Part model, mm, in its own coordinate system. A direction names the side the tool comes from. Round coordinates to 2 decimals unless told otherwise and drop trailing zeros. Write each loop counter-clockwise with the first axis right and the second up, starting at its lowest first coordinate (ties: lowest second). Pieces come first, ordered by that corner, then holes. Notation, with made-up numbers: (69.25, -13) -> (93.25, -13) arc R19 ccw to (93.25, 17) -> close; hole circle Ø1 at (20, 39). An arc over 180 degrees is marked (long way). Use CSV: the item, a comma, the result in double quotes. Start each with the question number.
(1) Saw through at D-D (x = -0.25). Give the cut face in (y, z).
(2) Saw through at A-A (x = 7.5). Give the cut face in (y, z), plus the area to 3 significant figures.
(3) Saw through at B-B (z = 0). Give the cut face in (x, y), plus the area to 3 significant figures.
(4) Which spindle directions (+Z, -Z, +X, -X, +Y, -Y) get a long thin tool onto all of the face, cutting with end or side? Do faces 5 (the flat face through (-11.5, 0.3, -4.3)), 6 (the flat face through (-12.5, 0.5, 0.1)). Say none if no direction does.
(5) Two-plate mould, pull along X, no slides. Class faces 1 (the cylindrical face through (-12.215, 0.507, 4.699)), 2 (the flat face through (-10, 0.3, -4.3)), 3 (the flat face through (10, 0.3, -4.3)), 4 (the flat face through (12.5, 0.5, -0.1)): released by +X, released by -X, zero draft, split by the parting line, or undercut.
(6) Probe line 1 (X direction, y = 0.65, z = 0); line 2 (Z direction, x = 7.5, y = 1.05); line 3 (X direction, y = 1.55, z = 0). List the from-to ranges inside material, lowest first. Write a range as [from, to].
Autodesk Inventor part; units mm, degrees
ref_plane "Work Plane1" through (0, 5, 0) normal (0, -1, 0) x (1, 0, 0)
ref_plane "YZ Plane" through (0, 0, 0) normal (1, 0, 0) x (0, 1, 0)
ref_plane "XZ Plane" through (0, 0, 0) normal (0, 1, 0) x (-1, 0, 0)
sketch "Sketch1" plane through (0, 0, 0) normal (0, 1, 0) x (-1, 0, 0)
  line L0 (12.5, -5) -> (-12.5, -5)
  line L1 (-12.5, -5) -> (-12.5, 5)
  line L2 (-12.5, 5) -> (12.5, 5)
  line L3 (12.5, 5) -> (12.5, -5)
  point P0 (0, 0)
  point P1 (12.5, 0)
  point P2 (0, -5)
  dimension "d0" = 10
  dimension "d2" = 25
extrude "Extrusion1" add sketch "Sketch1" along normal blind 2
sketch "Sketch2" plane through (0, 2, 0) normal (0, 1, 0) x (1, 0, 0)
  line L0 (12.5, 5) -> (-12.5, 5)
  line L1 (-12.5, 5) -> (-12.5, -5)
  line L2 (-12.5, -5) -> (12.5, -5)
  line L3 (0, 5) -> (0, -5) construction
  point P0 (0, 0)
  point P1 (-7.5, 0)
  point P2 (7.5, 0)
  point P3 (0, 0)
  dimension "d5" = 5
hole "Hole1" at (-7.5, 2, 0) at (7.5, 2, 0) direction (0, -1, 0) diameter 2.013 end through all
ref_plane "Work Plane1" through (0, 5, 0) normal (0, -1, 0) x (1, 0, 0)
sketch "Sketch4" plane through (0, 5, 0) normal (0, -1, 0) x (1, 0, 0)
  line L0 (-11.5, -7) -> (-10, -7) construction
  line L1 (-10, -7) -> (-10, -2) construction
  line L2 (-10, -2) -> (-11.5, -2) construction
  line L3 (-11.5, -2) -> (-11.5, -7) construction
  line L4 (-11.5, -7) -> (-10, -7)
  line L5 (-10, -7) -> (-10, -12)
  line L6 (-10, -12) -> (-11.5, -12)
  line L7 (-11.5, -12) -> (-11.5, -7)
  line L8 (12.5, -5) -> (-12.5, -5)
  line L9 (-12.5, -5) -> (-12.5, 5)
  line L10 (-12.5, -2) -> (-10, -2)
  point P0 (0, 0)
  dimension "d15" = 3
  dimension "d16" = 5
  dimension "d17" = 5
  dimension "d18" = 1.5
  dimension "d19" = 1
revolve "Revolution1" cut sketch "Sketch4" angle 90 about axis through (-12.5, 5, -2) along (-1, 0, 0)
fillet "Fillet1" radius 1 8 edges at (0, 2, 5) (12.5, 1, 5) (-12.5, 1, 5) (12.5, 2, 0) (-12.5, 2, 0) (0, 2, -5) (-12.5, 1, -5) (12.5, 1, -5)
mirror "Mirror1" about plane through (0, 0, 0) normal (1, 0, 0) of "Revolution1"
properties part number "CableHolder02"
Answers:
1,outline,"(0, -5) -> (1, -5) arc R1 ccw to (2, -4) -> (2, 4) arc R1 ccw to (1, 5) -> (0, 5) -> close"
2,outline,"(0, -5) -> (1, -5) arc R1 ccw to (2, -4) -> (2, -1.01) -> (0, -1.01) -> close; (0, 1.01) -> (2, 1.01) -> (2, 4) arc R1 ccw to (1, 5) -> (0, 5) -> close"
2,area,"15.5 mm²"
3,outline,"(-12.5, 0) -> (-8.51, 0) -> (-8.51, 2) -> (-11.5, 2) arc R1 ccw to (-12.5, 1) -> close; (-6.49, 0) -> (6.49, 0) -> (6.49, 2) -> (-6.49, 2) -> close; (8.51, 0) -> (12.5, 0) -> (12.5, 1) arc R1 ccw to (11.5, 2) -> (8.51, 2) -> close"
3,area,"41.5 mm²"
4,face 5,"-Z, -Y"
4,face 6,"+Z, -Z, -X, +Y, -Y"
5,face 1,"released by -X"
5,face 2,"undercut"
5,face 3,"undercut"
5,face 4,"released by +X"
6,line 1,"x = [-12.5, -8.51], [-6.49, 6.49], [8.51, 12.5]"
6,line 2,"z = [-5, -1.01], [1.01, 5]"
6,line 3,"x = [-12.34, -8.51], [-6.49, 6.49], [8.51, 12.34]"
